Model file for the job. Use its own axes, mm. Round coordinates to 2 decimals unless told otherwise and drop trailing zeros. Order: outer loops, then holes, each group sorted by start corner. A loop starts at its lowest first (then second) coordinate and runs counter-clockwise, first axis right, second up. Notation, with made-up numbers: (72, -7) -> (100, -7) arc R17 ccw to (100, 16) -> close; hole circle Ø5 at (25, 9.5). An arc over 180 degrees is marked (long way). Answer as CSV lines item,"result".
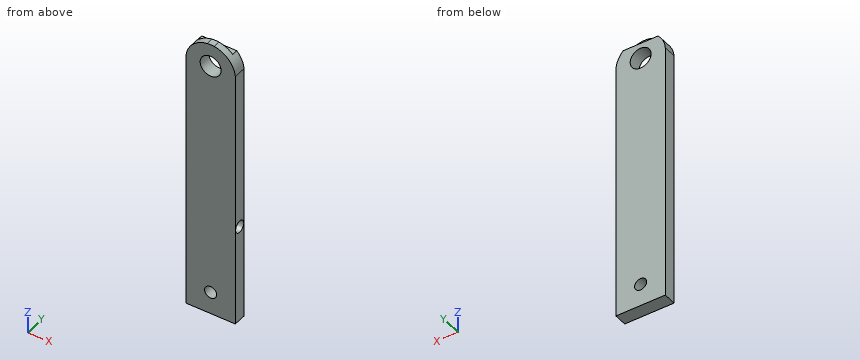
```python
from build123d import *

# Parameters (mm, degrees)
F0_R     = 2.7
F1_DEPTH = 3.33
F3_W     = 16.370755
F3_H     = 3.245242
F4_DEPTH = 1.52
F5_R     = 1.55
F6_DEPTH = 3.331
F7_R     = 1.55
F8_DEPTH = 5


with BuildPart() as f1:
    # F0 (on Front) → F1 (new body)
    with BuildSketch(Plane.XZ):
        with BuildLine():
            Line((0, 67.59), (0, 0))
            Line((0, 0), (12.75, 0))
            Line((12.75, 0), (12.75, 67.59))
            ThreePointArc((12.75, 67.59), (11.037405, 71.448822), (7.293558, 73.4))
            Line((7.293558, 73.4), (5.456442, 73.4))
            ThreePointArc((5.456442, 73.4), (1.712595, 71.448822), (0, 67.59))
        make_face()
        with Locations((6.375, 67.59)):
            Circle(F0_R, mode=Mode.SUBTRACT)
        with BuildLine():
            ThreePointArc((7.293558, 73.4), (6.375, 73.466301), (5.456442, 73.4))
            Line((5.456442, 73.4), (7.293558, 73.4))
        make_face()
    extrude(amount=F1_DEPTH)

    # F3 (on face) → F4 (cut)
    with BuildSketch(Plane(origin=(0, 0, 0), x_dir=(-1, 0, 0), z_dir=(0, 1, 0))):
        with Locations((-6.359821, 73.257189)):
            Rectangle(F3_W, F3_H)
    extrude(amount=-F4_DEPTH, mode=Mode.SUBTRACT)

    # F5 (on face) → F6 (cut, through all)
    with BuildSketch(Plane.XZ.offset(3.33)):
        with Locations((6.375, 5.81)):
            Circle(F5_R)
    extrude(amount=-F6_DEPTH, mode=Mode.SUBTRACT)

    # F7 (on face) → F8 (cut)
    with BuildSketch(Plane.YZ.offset(12.75)):
        with Locations((-1.665, 25.523206)):
            Circle(F7_R)
    extrude(amount=-F8_DEPTH, mode=Mode.SUBTRACT)


solid = f1.part
```
Q1. Flat gauge pins, fed straight in: pin 1 (1.5 mm diameter, centred on x = 5, z = 73, fed in from +Y); pin 2 (0.5 mm diameter, centred on x = 8.5, y = -0.5, fed in from +Z). Where does each tip first touch, or does it go through?
Checks:
pin 1,"y = -1.52"
pin 2,"z = 71.63"
Q2. Saw through at B-B (y = -2.5). Write the cut outline in (x, z) (3 decimals).
Checks:
outline,"(0, 0) -> (12.75, 0) -> (12.75, 24.217) -> (7.75, 24.217) -> (7.75, 26.829) -> (12.75, 26.829) -> (12.75, 67.59) arc R6.396 ccw to (7.294, 73.4) arc R6.396 ccw to (5.456, 73.4) arc R6.396 ccw to (0, 67.59) -> close; hole circle Ø5.4 at (6.375, 67.59); hole circle Ø3.1 at (6.375, 5.81)"
Q3. Saw through at A-A (z = 5.81). Write the cut outline in (x, y) (3 decimals), plus the area to 3 significant figures.
Checks:
outline,"(0, -3.33) -> (4.825, -3.33) -> (4.825, 0) -> (0, 0) -> close; (7.925, -3.33) -> (12.75, -3.33) -> (12.75, 0) -> (7.925, 0) -> close"
area,"32.1 mm²"
Q4. Wall check: L1, parallel to Z at x = 6.25, y = -1.2; L2, parallel to Z at x = 5.5, y = -2.8; L3, parallel to Z at x = 10, y = -1.45. Give the ranges that are in metal, low to high. Write a range as [from, to].
Checks:
L1,"[0, 4.27], [7.35, 64.89], [70.29, 71.63]"
L2,"[0, 4.53], [7.09, 65.04], [70.14, 73.41]"
L3,"[0, 23.99], [27.06, 71.63]"
